Design review of the part shown in the three views and the two pictorial views. Dimensions are in mm from the part's minimum x, y and z. A direction names the side the tool comes from. Coordinates: 2 decimals unless noted, no trailing zeros. Loops run counter-clockwise (first coordinate to the right, second up) from the corner with the lowest first, then second, coordinate; pieces in that order, holes last. Notation, with made-up numbers: M 19,-37 L 67,-37 A19 ccw 67,-1 Z; hole C 70,6 d8. An arc over 180 degrees is marked long. Put each result on its own line as item: value. Start each with the question number.
(1) For the marked faces 1 and 2, list the 3-axis set-ups (+Z, -Z, +X, -X, +Y, -Y) from which the entire face can be reached by the end or side of a thin tool; tool diameter is ignored.
(2) Clearance check with flat-ended pins moving along their axes: pin 1 (4 mm diameter, centred on x = 320.5, y = 10.5, fed in from -Z); pin 2 (10.5 mm diameter, centred on x = 870, z = 390, fed in from +Y). State where each tip first meets the part, or that it passes through.
(3) Take a section at A-A, the plane x = 294. Give the boundary of the cut face in (y, z).
(4) Take a section at B-B, the plane y = 4.25. Give the boundary of the cut face in (x, z), then the cut area to 3 significant figures.
(5) For probe 1 along X at (y, z) = (6, 390); probe 2 along Z at (x, y) = (870, 4.5); probe 3 along X at (y, z) = (2.5, 219.5), list the stretches that pass through material, from the lowest coordinate up. Write a range as [from, to].
(6) Take a section at C-C, the plane z = 370. Give the boundary of the cut face in (x, y).
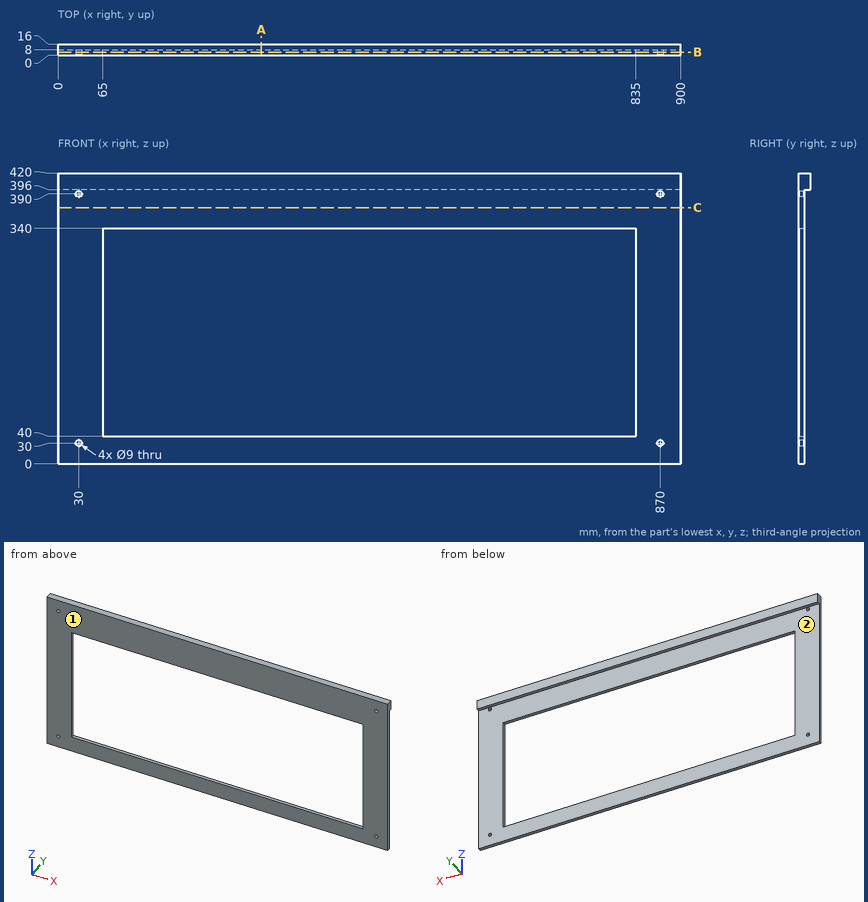
Computed values:
1. face 1: +Z, -Z, +X, -X, -Y
1. face 2: -Z, +X, -X, +Y
2. pin 1: stops at z = 396
2. pin 2: stops at y = 8
3. outline: M 0,0 L 8,0 L 8,40 L 0,40 Z; M 0,340 L 8,340 L 8,396 L 16,396 L 16,420 L 0,420 Z
4. outline: M 0,0 L 900,0 L 900,420 L 0,420 Z; hole C 30,30 d9; hole C 30,390 d9; hole M 65,40 L 835,40 L 835,340 L 65,340 Z; hole C 870,30 d9; hole C 870,390 d9
4. area: 147,000 mm^2
5. probe 1: x = [0, 25.5], [34.5, 865.5], [874.5, 900]
5. probe 2: z = [0, 25.5], [34.5, 385.5], [394.5, 420]
5. probe 3: x = [0, 65], [835, 900]
6. outline: M 0,0 L 900,0 L 900,8 L 0,8 Z
